Read the model definition and answer for the solid it produces. Units are mm, in the model's axes. Face numbers are marked on the shaded views. Give positions to 0.01 mm unless a question says otherwise; leave off trailing zeros. Order: outer loops, then holes, each group sorted by start corner. A loop starts at its lowest first (then second) coordinate and runs counter-clockwise, first axis right, second up. Notation, with made-up numbers: (6.25, -37.5) - (10.25, -37.5) arc R20 ccw to (10.25, -17.5) - close; hole circle Ø11 at (19, 79). An arc over 180 degrees is marked (long way). Write item = value, one per line.
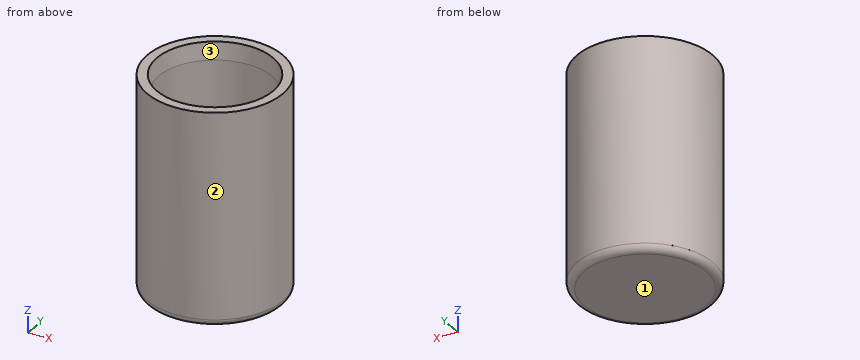
```python
from build123d import *

# Parameters (mm, degrees)
F0_R     = 19.5140017551
F0_R_2   = 16.2285581311
F1_DEPTH = 2
F2_DEPTH = 59
F4_SIZE2 = 0.5
F4_SIZE  = 5


# Not quite as in the source:
# - a fillet or chamfer that OpenCascade refuses, or shapes differently, is made with other operations: its cross-section is extruded or revolved along the edge and cut away or added


with BuildPart() as f1:
    # F0 (on Top) → F1 (new body)
    with BuildSketch(Plane.XY):
        Circle(F0_R)
        Circle(F0_R_2, mode=Mode.SUBTRACT)
        Circle(F0_R_2)
    extrude(amount=-F1_DEPTH)

    # F0 (on Top) → F2 (join)
    with BuildSketch(Plane.XY):
        Circle(F0_R)
        Circle(F0_R_2, mode=Mode.SUBTRACT)
    extrude(amount=F2_DEPTH)

    # F3: fillet of radius 2 on 2 edges, made by hand

    # F3_s1 → F3_t2 (revolve, cut)
    with BuildSketch(Plane.XZ):
        with BuildLine():
            ThreePointArc((19.5140017551, 0), (18.9282153175, -1.4142135624), (17.5140017551, -2))
            Line((17.5140017551, -2), (19.5140017551, -2))
            Line((19.5140017551, -2), (19.5140017551, 0))
        make_face()
    revolve(axis=Axis((0, 0, -2), (0, 0, 1)), mode=Mode.SUBTRACT)

    # F3_s3 → F3_t4 (revolve)
    with BuildSketch(Plane.XZ):
        with BuildLine():
            ThreePointArc((16.2285581311, 2), (15.6427716934, 0.5857864376), (14.2285581311, 0))
            Line((14.2285581311, 0), (16.2285581311, 0))
            Line((16.2285581311, 0), (16.2285581311, 2))
        make_face()
    revolve(axis=Axis((0, 0, 0), (0, 0, 1)))

    # F4
    f4_edges = [f1.edges().sort_by_distance(p)[0] for p in [
        (-16.228558, 0, 59),
    ]]
    f4_side = f1.faces().sort_by_distance((-16.228558, 0, 30.5))[0]
    chamfer(f4_edges, length=F4_SIZE, length2=F4_SIZE2, reference=f4_side)


solid = f1.part
```
1. Determine the mould class of the marked faces 1, 2 and 3 for opening direction Y: +Y half, -Y half, draft (parallel to the pull), parting line (faces both ways), or undercut.
Recorded:
face_1 = draft
face_2 = parting line
face_3 = undercut
2. Flat-ended cylindrical pins translate along their axes: pin 1 (4 mm diameter, centred on y = 3, z = 48, fed in from +X); pin 2 (1.5 mm diameter, centred on x = 12, y = -11, fed in from +Z); pin 3 (23 mm diameter, centred on x = 2, y = -2.5, fed in from +Z); pin 4 (6 mm diameter, centred on x = 8, y = 1, fed in from +Z). Find the tip coordinate at first contact, or state that the pin passes through.
Recorded:
pin_1 = 19.49
pin_2 = 59
pin_3 = 0.06
pin_4 = 0
3. Straight lines are drawn through the part: L1, parallel to Y at x = 0, z = 21; L2, parallel to Z at x = -5, y = 13.5; L3, parallel to X at y = -13, z = 54.5. For each, find the intervals that lie inside material, in ascending order. Write a range as [from, to].
Recorded:
L1 = [-19.51, -16.23], [16.23, 19.51]
L2 = [-2, 0.01]
L3 = [-14.55, -9.8], [9.8, 14.55]
4. Section A-A (y = 0) is taken. Determine the outline of the cut face in (x, z).
Recorded:
outline = (-19.51, 0) arc R2 ccw to (-17.51, -2) - (17.51, -2) arc R2 ccw to (19.51, 0) - (19.51, 59) - (16.73, 59) - (16.23, 54) - (16.23, 2) arc R2 cw to (14.23, 0) - (-14.23, 0) arc R2 cw to (-16.23, 2) - (-16.23, 54) - (-16.73, 59) - (-19.51, 59) - close
5. Section C-C (z = 29.5) is taken. Determine the outline of the cut face in (x, y), and give its area (3 significant figures).
Recorded:
outline = circle Ø39.03 at (0, 0); hole circle Ø32.46 at (0, 0)
area = 369 mm^2
